Job drawing, mm, ordinate dimensions from the low corner. One solid piece. Give positions to 0.01 mm unless a question says otherwise; leave off trailing zeros. Write each loop counter-clockwise with the first axis right and the second up, starting at its lowest first coordinate (ties: lowest second). Pieces come first, ordered by that corner, then holes. Notation, with made-up numbers: M 65.5,78.5 L 83.5,78.5 A8 ccw 83.5,85.5 Z; hole C 60.5,-38.75 d4. An arc over 180 degrees is marked long. Answer as CSV lines item,"result". Start each with the question number.
1) Slice it at B-B, the plane z = 4.75. Give the cut face in (x, y), plus the area to 3 significant figures.
2) Slice it at D-D, the plane x = 31. Give the cut face in (y, z), plus the area to 3 significant figures.
3) Slice it at C-C, the plane y = 18. Give the cut face in (x, z), plus the area to 3 significant figures.
4) Slice it at A-A, the plane x = 72.5. Give the cut face in (y, z), plus the area to 3 significant figures.
5) Pin check, flat tips, straight feed: pin 1 Ø1.5 at (x, z) = (106.5, 4.5) entering from -Y; pin 2 Ø5.5 at (x, y) = (38.5, 7) entering from -Z; pin 3 Ø4 at (x, z) = (18, 4) entering from +Y. Stop position of each tip, or through.
6) Wall check: line 1 along Y through (x, z) = (69, 7.75); line 2 along X through (y, z) = (32.5, 8.5); line 3 along Y through (x, z) = (102, 5). Give the ranges that are in metal, low to high. Write a range as from..to.
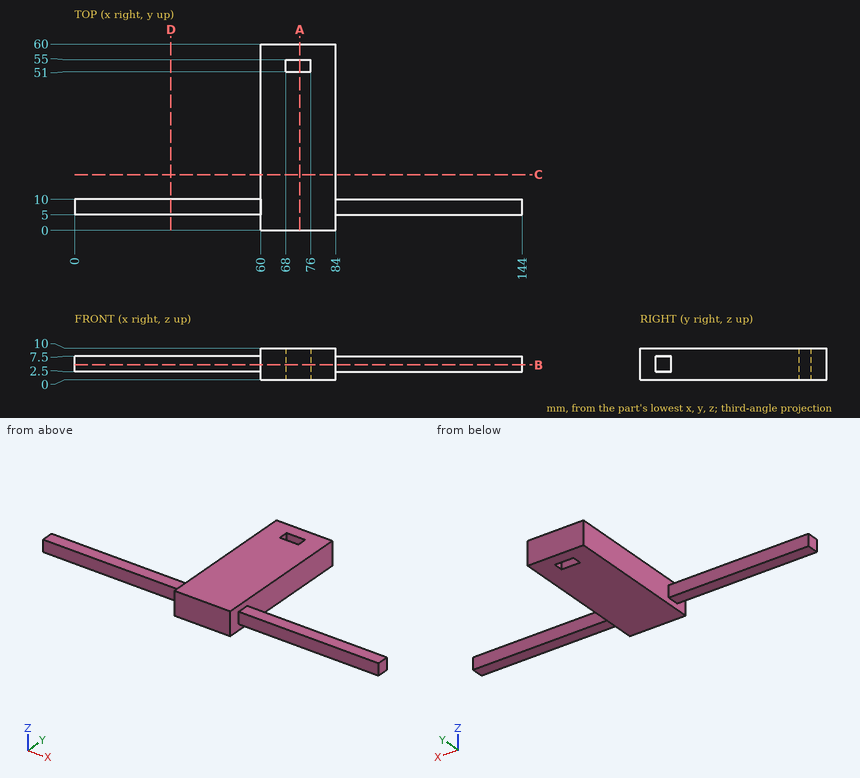
Found:
1,outline,"M 0,5 L 60,5 L 60,0 L 84,0 L 84,5 L 144,5 L 144,10 L 84,10 L 84,60 L 60,60 L 60,10 L 0,10 Z; hole M 68,51 L 76,51 L 76,55 L 68,55 Z"
1,area,"2,010 mm²"
2,outline,"M 5,2.5 L 10,2.5 L 10,7.5 L 5,7.5 Z"
2,area,"25.0 mm²"
3,outline,"M 60,0 L 84,0 L 84,10 L 60,10 Z"
3,area,"240 mm²"
4,outline,"M 0,0 L 51,0 L 51,10 L 0,10 Z; M 55,0 L 60,0 L 60,10 L 55,10 Z"
4,area,"560 mm²"
5,pin 1,"y = 5"
5,pin 2,"z = 2.5"
5,pin 3,"y = 10"
6,line 1,"0..51, 55..60"
6,line 2,"60..84"
6,line 3,"5..10"
